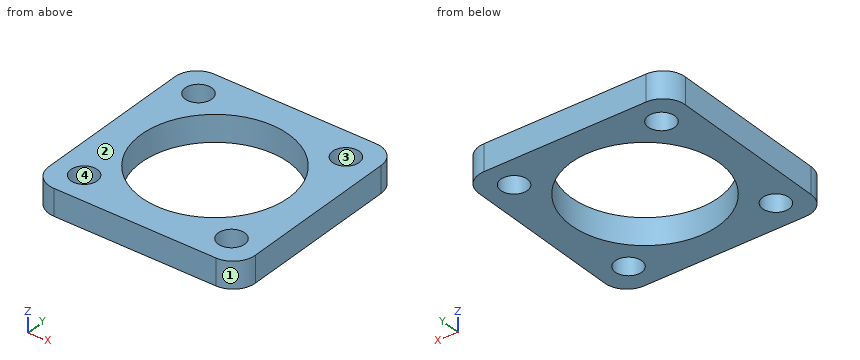
from build123d import *

# Parameters (mm, degrees)
F0_W     = 140
F0_H     = 140
F1_DEPTH = 18
F2_R     = 15
F4_D     = 18
F5_R     = 50
F6_DEPTH = 18.001


with BuildPart() as f1:
    # F0 (on Top) → F1 (new body)
    with BuildSketch(Plane.XY):
        with Locations((70, -70)):
            Rectangle(F0_W, F0_H)
    extrude(amount=F1_DEPTH)

    # F2
    f2_edges = [f1.edges().sort_by_distance(p)[0] for p in [
        (0, -140, 9),
        (140, -140, 9),
        (140, 0, 9),
        (0, 0, 9),
    ]]
    fillet(f2_edges, radius=F2_R)

    # F4 (through all)
    with Locations(Plane.XY.offset(18)):
        with Locations((120, -120), (20, -120), (20, -20), (120, -20)):
            Hole(F4_D / 2)

    # F5 (on face) → F6 (cut, through all)
    with BuildSketch(Plane.XY.offset(18)):
        with Locations((70, -70)):
            Circle(F5_R)
    extrude(amount=-F6_DEPTH, mode=Mode.SUBTRACT)


solid = f1.part
Could you check a few things on this model? Use its own coordinates, in mm. Face numbers are marked on the shaded views. Round coordinates to 2 decimals unless told otherwise and drop trailing zeros. Write each loop counter-clockwise with the first axis right and the second up, starting at its lowest first coordinate (ties: lowest second). Pieces come first, ordered by that corner, then holes. Notation, with made-up numbers: (27, -1) - (69, -1) arc R14 cw to (69, 15) - close; hole circle Ø3 at (-7.5, 35). An arc over 180 degrees is marked (long way). Put each result on its own line as item: value. Start each with the question number.
(1) I want a section at D-D, the plane y = -56.5. Please give me the cut outline in (x, z).
(2) I want a section at B-B, the plane z = 6.75. Please give me the cut outline in (x, y), plus the area to 3 significant figures.
(3) I need wall thicknesses on probe 1 along X at (y, z) = (-12.5, 6.25); probe 2 along X at (y, z) = (-77.5, 10); probe 3 along Y at (x, z) = (68.5, 12.25). Which ranges of each line are inside material? Lowest first, please.
(4) Thinking about a two-plate mould opening in X: for the marked faces 1, 2, 3 and 4, which applies, released by +X, released by -X, zero draft, split by the parting line, or undercut?
(5) I want a section at C-C, the plane y = -24.5. Please give me the cut outline in (x, z).
(6) I want a section at A-A, the plane x = 84. Please give me the cut outline in (y, z).
Here are the results:
1. outline: (0, 0) - (21.86, 0) - (21.86, 18) - (0, 18) - close; (118.14, 0) - (140, 0) - (140, 18) - (118.14, 18) - close
2. outline: (0, -125) arc R15 ccw to (15, -140) - (125, -140) arc R15 ccw to (140, -125) - (140, -15) arc R15 ccw to (125, 0) - (15, 0) arc R15 ccw to (0, -15) - close; hole circle Ø18 at (20, -120); hole circle Ø18 at (20, -20); hole circle Ø100 at (70, -70); hole circle Ø18 at (120, -120); hole circle Ø18 at (120, -20)
2. area: 10,500 mm^2
3. probe 1: x = 0.21 to 15.03, 24.97 to 115.03, 124.97 to 139.79
3. probe 2: x = 0 to 20.57, 119.43 to 140
3. probe 3: y = -140 to -119.98, -20.02 to 0
4. face 1: released by +X
4. face 2: zero draft
4. face 3: undercut
4. face 4: undercut
5. outline: (0, 0) - (12.21, 0) - (12.21, 18) - (0, 18) - close; (27.79, 0) - (49.27, 0) - (49.27, 18) - (27.79, 18) - close; (90.73, 0) - (112.21, 0) - (112.21, 18) - (90.73, 18) - close; (127.79, 0) - (140, 0) - (140, 18) - (127.79, 18) - close
6. outline: (-140, 0) - (-118, 0) - (-118, 18) - (-140, 18) - close; (-22, 0) - (0, 0) - (0, 18) - (-22, 18) - close
